```python
from build123d import *

# Parameters (mm, degrees)
F0_W     = 800
F0_H     = 80
F1_DEPTH = 40
F0_W_2   = 420
F0_W_3   = 80
F0_H_2   = 538.2458400726
F2_DEPTH = 40
F3_DEPTH = 40


# Not quite as in the source:
# - a feature names something its author has since deleted; it is built from what else it names


with BuildPart() as f1:
    # F0 (on Front) → F1 (new body)
    with BuildSketch(Plane.XZ):
        with Locations((400, 1800)):
            Rectangle(F0_W, F0_H)
        Polygon((-80, 1840), (-80, -80), (0, -80), (0, 0), (0, 538.2458400726), (0, 618.2458400726), (0, 1760), (0, 1840), align=None)
        with Locations((400, -40)):
            Rectangle(F0_W, F0_H)
        Polygon((800, 0), (800, -80), (880, -80), (880, 0), (880, 538.2458400726), (880, 618.2458400726), (880, 1840), (800, 1840), (800, 1760), (800, 618.2458400726), (800, 538.2458400726), align=None)
    extrude(amount=F1_DEPTH)

    # F0 (on Front) → F2 (join)
    with BuildSketch(Plane.XZ):
        Polygon((-80, 1840), (-80, -80), (0, -80), (0, 0), (0, 538.2458400726), (0, 618.2458400726), (0, 1760), (0, 1840), align=None)
        with Locations((400, -40)):
            Rectangle(F0_W, F0_H)
        with Locations((400, 1800)):
            Rectangle(F0_W, F0_H)
        Polygon((800, 0), (800, -80), (880, -80), (880, 0), (880, 538.2458400726), (880, 618.2458400726), (880, 1840), (800, 1840), (800, 1760), (800, 618.2458400726), (800, 538.2458400726), align=None)
        Polygon((880, 0), (880, -80), (1380, -80), (1380, 0), (1300, 0), align=None)
        with Locations((1090, 578.2458400726)):
            Rectangle(F0_W_2, F0_H)
        with Locations((1340, 269.1229200363)):
            Rectangle(F0_W_3, F0_H_2)
        with Locations((1340, 578.2458400726)):
            Rectangle(F0_W_3, F0_H)
    extrude(amount=F2_DEPTH)

    # F0 (on Front) → F3 (join)
    with BuildSketch(Plane.XZ):
        with Locations((400, 578.2458400726)):
            Rectangle(F0_W, F0_H)
    extrude(amount=F3_DEPTH)


solid = f1.part
```
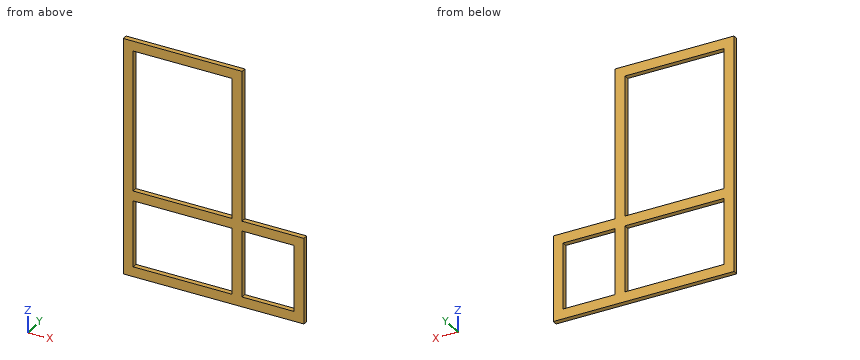
Design review of the part built by this model. Coordinates are the model's own, in mm. Coordinates: 2 decimals unless noted, no trailing zeros. Loops run counter-clockwise (first coordinate to the right, second up) from the corner with the lowest first, then second, coordinate; pieces in that order, holes last. Notation, with made-up numbers: (77, 55.25) -> (133, 55.25) arc R17 cw to (133, 79.25) -> close; hole circle Ø1 at (49, -39.5). An arc over 180 degrees is marked (long way). Answer as a JSON object with one key per item and string values.
Q1. Take a section at A-A on x = 108. Give the boundary of the cut face in (y, z).
Answer block:
{"outline": "(-40, -80) -> (0, -80) -> (0, 0) -> (-40, 0) -> close; (-40, 538.25) -> (0, 538.25) -> (0, 618.25) -> (-40, 618.25) -> close; (-40, 1760) -> (0, 1760) -> (0, 1840) -> (-40, 1840) -> close"}
Q2. Take a section at B-B on y = -28.5. Give the boundary of the cut face in (x, z), plus the area to 3 significant figures.
Answer block:
{"outline": "(-80, -80) -> (1380, -80) -> (1380, 618.25) -> (880, 618.25) -> (880, 1840) -> (-80, 1840) -> close; hole (0, 0) -> (800, 0) -> (800, 538.25) -> (0, 538.25) -> close; hole (0, 618.25) -> (800, 618.25) -> (800, 1760) -> (0, 1760) -> close; hole (880, 0) -> (1300, 0) -> (1300, 538.25) -> (880, 538.25) -> close", "area": "622,000 mm^2"}
Q3. Clearance check with flat-ended pins moving along their axes: pin 1 Ø4 at (x, y) = (1088, -14.5) entering from +Z; pin 2 Ø20 at (y, z) = (-11, 961.5) entering from +X. State where each tip first meets the part, or that it passes through.
Answer block:
{"pin 1": "stops at z = 618.25", "pin 2": "stops at x = 880"}
Q4. Take a section at C-C on z = 962. Give the boundary of the cut face in (x, y).
Answer block:
{"outline": "(-80, -40) -> (0, -40) -> (0, 0) -> (-80, 0) -> close; (800, -40) -> (880, -40) -> (880, 0) -> (800, 0) -> close"}
Q5. To check wall thickness, follow L1, parallel to X at y = -17, z = 404; L2, parallel to Z at x = 445, y = -9.5; L3, parallel to X at y = -12.5, z = 1620. State the ranges of each line that lie inside material, in increasing order.
Answer block:
{"L1": "x = -80 to 0, 800 to 880, 1300 to 1380", "L2": "z = -80 to 0, 538.25 to 618.25, 1760 to 1840", "L3": "x = -80 to 0, 800 to 880"}
